Check sheet for the modelled part. Datum: model origin and axes. Units: mm. A direction names the side the tool comes from. Round coordinates to 2 decimals unless told otherwise and drop trailing zeros. Order: outer loops, then holes, each group sorted by start corner. A loop starts at its lowest first (then second) coordinate and runs counter-clockwise, first axis right, second up. Notation, with made-up numbers: (-1.5, 12.25) -> (23.5, 12.25) arc R14 cw to (23.5, 26.25) -> close; hole circle Ø7 at (49, -19). An arc over 180 degrees is marked (long way). Answer in a Markdown table with one row per item.
Autodesk Fusion 360 part; units mm, degrees
sketch "草图1" plane through (0, 0, 0) normal (0, 0, 1) x (1, 0, 0)
  line L0 (0, 0) -> (60, 0)
  line L1 (60, 0) -> (60, -90)
  line L2 (60, -90) -> (0, -90)
  line L3 (0, -90) -> (0, 0)
  dimension "d1" = 60
  dimension "d2" = 90
extrude "拉伸1" add sketch "草图1" along normal blind 30
sketch "草图2" plane through (0, 0, 30) normal (0, 0, 1) x (-1, 0, 0)
  line L0 (0, 90) -> (-60, 90)
  line L1 (-60, 90) -> (-60, 0)
  line L2 (-60, 0) -> (0, 0)
  line L3 (0, 0) -> (0, 90)
  line L4 (-5, 5) -> (-55, 5)
  line L5 (-55, 5) -> (-55, 85)
  line L6 (-55, 85) -> (-5, 85)
  line L7 (-5, 85) -> (-5, 5)
  dimension "d5" = 50
  dimension "d6" = 80
  dimension "d7" = 55
  dimension "d8" = 5
extrude "拉伸2" cut sketch "草图2" against normal blind 25 contours L4 L5 L6 L7
sketch "草图3" plane through (0, -90, 0) normal (0, -1, 0) x (1, 0, 0)
  line L0 (0, 0) -> (60, 0)
  line L1 (60, 0) -> (60, 30)
  line L2 (60, 30) -> (0, 30)
  line L3 (0, 30) -> (0, 0)
sketch "草图4" plane through (0, 0, 5) normal (0, 0, 1) x (-1, 0, 0)
  line L0 (-5, 85) -> (-55, 85)
  line L1 (-55, 85) -> (-55, 5)
  line L2 (-55, 5) -> (-5, 5)
  line L3 (-5, 5) -> (-5, 85)
  circle A0 centre (-15.0278, 14.2331) radius 0.5
sketch "草图5" plane through (0, 0, 30) normal (0, 0, 1) x (-1, 0, 0)
  line L0 (-55, 5) -> (-55, 85)
  line L1 (-55, 85) -> (-5, 85)
  line L2 (-5, 85) -> (-5, 5)
  line L3 (-5, 5) -> (-55, 5)
  line L4 (0, 90) -> (-60, 90)
  line L5 (-60, 90) -> (-60, 0)
  line L6 (-60, 0) -> (0, 0)
  line L7 (0, 0) -> (0, 90)
  line L8 (-2.5, 2.5) -> (-57.5, 2.5)
  line L9 (-57.5, 2.5) -> (-57.5, 87.5)
  line L10 (-57.5, 87.5) -> (-2.5, 87.5)
  line L11 (-2.5, 87.5) -> (-2.5, 2.5)
  dimension "d12" = 55
  dimension "d13" = 85
  dimension "d14" = 2.5
  dimension "d15" = 87.5
extrude "拉伸3" add sketch "草图5" along normal blind 3 contours L8 L9 L10 L11
(1) Section check B-B on y = -55. Record the boundary of the cut face in (x, z).
Solutions:
| item | result |
|---|---|
| outline | (0, 0) -> (60, 0) -> (60, 30) -> (57.5, 30) -> (57.5, 33) -> (55, 33) -> (55, 5) -> (5, 5) -> (5, 33) -> (2.5, 33) -> (2.5, 30) -> (0, 30) -> close |
(2) Depth check by flat-ended pin: pin 1 Ø1.5 at (y, z) = (-49, 31.5) entering from -X; pin 2 Ø2.5 at (x, z) = (29, 32) entering from -Y; pin 3 Ø1.5 at (x, y) = (33.5, -29.5) entering from +Z. Enter the tip coordinate at first touch or a pass-through.
Solutions:
| item | result |
|---|---|
| pin 1 | x = 2.5 |
| pin 2 | y = -87.5 |
| pin 3 | z = 5 |
(3) Section check C-C on x = 10. Record the boundary of the cut face in (y, z), plus the area to 3 significant figures.
Solutions:
| item | result |
|---|---|
| outline | (-90, 0) -> (0, 0) -> (0, 30) -> (-2.5, 30) -> (-2.5, 33) -> (-5, 33) -> (-5, 5) -> (-85, 5) -> (-85, 33) -> (-87.5, 33) -> (-87.5, 30) -> (-90, 30) -> close |
| area | 715 mm^2 |
(4) Tool access check on faces 4 (the flat face through (30, -2.5, 31)), 5 (the flat face through (30, -87.5, 31)), 6 (the flat face through (57.5, -44, 31)), 7 (the flat face through (30, -85, 19)). Record the directions out of +Z, -Z, +X, -X, +Y, -Y that give a thin tool (end or side, any length) a straight path to the whole face; none if there is none.
Solutions:
| item | result |
|---|---|
| face 4 | +Z, +X, -X, +Y |
| face 5 | +Z, +X, -X, -Y |
| face 6 | +Z, +X, +Y, -Y |
| face 7 | +Z |
(5) Section check A-A on z = 14.5. Record the boundary of the cut face in (x, y).
Solutions:
| item | result |
|---|---|
| outline | (0, -90) -> (60, -90) -> (60, 0) -> (0, 0) -> close; hole (5, -85) -> (55, -85) -> (55, -5) -> (5, -5) -> close |
(6) Scan lines: probe 1 along Y at (x, z) = (37.5, 23); probe 2 along X at (y, z) = (-28.5, 14.5); probe 3 along Z at (x, y) = (24, -68.5). Record each from-to range of solid material in increasing order. Write a range as from..to.
Solutions:
| item | result |
|---|---|
| probe 1 | -90..-85, -5..0 |
| probe 2 | 0..5, 55..60 |
| probe 3 | 0..5 |
(7) Draft check along X on faces 1 (the flat face through (30, -5, 19)), 2 (the flat face through (30, -90, 15)), 3 (the flat face through (60, -44, 15)). Enter one of: pulls with the +X half, pulls with the -X half, needs draft (parallel to the pull), parting line crosses it, or undercut.
Solutions:
| item | result |
|---|---|
| face 1 | undercut |
| face 2 | needs draft |
| face 3 | pulls with the +X half |
